The listing builds one solid part. Answer for the finished solid, in the listing's coordinates (mm). Give positions to 0.01 mm unless a question says otherwise; leave off trailing zeros. Write each loop counter-clockwise with the first axis right and the second up, starting at its lowest first coordinate (ties: lowest second). Pieces come first, ordered by that corner, then holes. Notation, with made-up numbers: M -7,28 L 26,28 A12 cw 26,36 Z; hole C 65.5,23 d5. An arc over 180 degrees is marked long. Answer as a JSON object with one key per item and string values.
```python
from build123d import *

# Parameters (mm, degrees)
BOSS_EXTRUDE1_DEPTH = 330.2
BOSS_EXTRUDE2_DEPTH = 0.254


with BuildPart() as part:
    # Sketch1 → Boss-Extrude1 (new body)
    with BuildSketch(Plane(origin=(0, 0, 0), x_dir=(1, 0, 0), z_dir=(0, 1, 0))):
        Polygon((0, 0), (-143.684097937, -143.684097937), (-161.644610179, -125.723585695), (-14.368409794, 21.552614691), (147.276200386, -140.091995489), (143.684097937, -143.684097937), align=None)
    extrude(amount=BOSS_EXTRUDE1_DEPTH)

    # Sketch2 → Boss-Extrude2 (add)
    with BuildSketch(Plane(origin=(0, 0, 0), x_dir=(0.707106781, 0, -0.707106781), z_dir=(0.707106781, 0, 0.707106781))):
        Polygon((0, 330.2), (0, 127), (-203.2, 127), align=None)
    extrude(amount=BOSS_EXTRUDE2_DEPTH)


solid = part.part
```
1. A cutting plane is placed at D-D, the plane z = 38. Give the vertices of the cut face in (x, y), plus the area to 3 significant figures.
Verdict:
{"outline": "M -73.92,0 L -38,0 L -38,127 L -37.64,127 L -37.64,276.71 L -38,276.46 L -38,330.2 L -73.92,330.2 Z; M 38,0 L 45.18,0 L 45.18,330.2 L 38,330.2 Z", "area": "14,300 mm2"}
2. A cutting plane is placed at B-B, the plane y = 26. Give the vertices of the cut face in (x, z), plus the area to 3 significant figures.
Verdict:
{"outline": "M -161.64,125.72 L -14.37,-21.55 L 147.28,140.09 L 143.68,143.68 L 0,0 L -143.68,143.68 Z", "area": "6,320 mm2"}
3. A cutting plane is placed at A-A, the plane z = 130. Give the vertices of the cut face in (x, y), plus the area to 3 significant figures.
Verdict:
{"outline": "M -157.37,0 L -130,0 L -130,127 L -129.64,127 L -129.64,146.61 L -130,146.35 L -130,330.2 L -157.37,330.2 Z; M 130,0 L 137.18,0 L 137.18,330.2 L 130,330.2 Z", "area": "11,400 mm2"}
4. Flat-ended cylindrical pins translate along their axes: pin 1 (3 mm diameter, centred on x = -119, y = 173.5, fed in from +Z); pin 2 (5 mm diameter, centred on x = 6, y = 210.5, fed in from +Z); pin 3 (6 mm diameter, centred on x = 60, y = 168, fed in from -Z). Find the tip coordinate at first contact, or state that the pin passes through.
Verdict:
{"pin 1": "stops at z = 120.5", "pin 2": "stops at z = 8.5", "pin 3": "stops at z = 49.82"}
5. The mould has two halves that part along X. Classify faces 1 (the flat face through (-64, 330.2, 61)), 2 (the flat face through (65.322, 162.789, 58.138)), 3 (the flat face through (-38.73, 184.87, 39.09)): released by +X, released by -X, zero draft, split by the parting line, or undercut.
Verdict:
{"face 1": "zero draft", "face 2": "released by +X", "face 3": "undercut"}
6. Consider line 1 along X through (y, z) = (165, 98.5); line 2 along X through (y, z) = (23, 95); line 3 along Z through (x, y) = (-12, 182). Determine where each line is inside the solid, lowest interval first.
Verdict:
{"line 1": "x = -134.42 to -98.14, 98.5 to 105.68", "line 2": "x = -130.92 to -95, 95 to 102.18", "line 3": "z = -19.18 to 12.36"}
7. A cutting plane is placed at C-C, the plane x = -19. Give the vertices of the cut face in (y, z), plus the area to 3 significant figures.
Verdict:
{"outline": "M 0,-16.92 L 330.2,-16.92 L 330.2,19 L 303.33,19 L 303.08,19.36 L 127,19.36 L 127,19 L 0,19 Z", "area": "11,900 mm2"}
